```python
from build123d import *

# Parameters (mm, degrees)
SKETCH1_R           = 62.5
BOSS_EXTRUDE1_DEPTH = 25
SKETCH3_W           = 40
SKETCH3_H           = 21
SKETCH7_R           = 6.05
CUT_EXTRUDE1_DEPTH  = 205.205778567
SCALE1_SCALE        = 0.25


with BuildPart() as part:
    # Sketch1 → Boss-Extrude1 (new, symmetric)
    with BuildSketch(Plane(origin=(0, 0, 0), x_dir=(1, 0, 0), z_dir=(0, 1, 0))):
        with BuildLine():
            Line((102.443626017, 46.492510026), (95.514529523, 43.622384283))
            Line((95.514529523, 43.622384283), (98.384655266, 36.693287789))
            Line((98.384655266, 36.693287789), (105.31375176, 39.563413532))
            ThreePointArc((105.31375176, 39.563413532), (110.313875085, 22.070318614), (112.4288664, 4))
            Line((112.4288664, 4), (140, 4))
            Line((140, 4), (140, -4))
            Line((140, -4), (112.4288664, -4))
            ThreePointArc((112.4288664, -4), (110.313875085, -22.070318614), (105.31375176, -39.563413532))
            Line((105.31375176, -39.563413532), (98.384655266, -36.693287789))
            Line((98.384655266, -36.693287789), (95.514529523, -43.622384283))
            Line((95.514529523, -43.622384283), (102.443626017, -46.492510026))
            ThreePointArc((102.443626017, -46.492510026), (93.609761087, -62.397617177), (82.327640957, -76.670786708))
            Line((82.327640957, -76.670786708), (101.823376491, -96.166522241))
            Line((101.823376491, -96.166522241), (96.166522241, -101.823376491))
            Line((96.166522241, -101.823376491), (76.670786708, -82.327640957))
            ThreePointArc((76.670786708, -82.327640957), (62.397617177, -93.609761087), (46.492510026, -102.443626017))
            Line((46.492510026, -102.443626017), (43.622384283, -95.514529523))
            Line((43.622384283, -95.514529523), (36.693287789, -98.384655266))
            Line((36.693287789, -98.384655266), (39.563413532, -105.31375176))
            ThreePointArc((39.563413532, -105.31375176), (22.070318614, -110.313875085), (4, -112.4288664))
            Line((4, -112.4288664), (4, -140))
            Line((4, -140), (-4, -140))
            Line((-4, -140), (-4, -112.4288664))
            ThreePointArc((-4, -112.4288664), (-22.070318614, -110.313875085), (-39.563413532, -105.31375176))
            Line((-39.563413532, -105.31375176), (-36.693287789, -98.384655266))
            Line((-36.693287789, -98.384655266), (-43.622384283, -95.514529523))
            Line((-43.622384283, -95.514529523), (-46.492510026, -102.443626017))
            ThreePointArc((-46.492510026, -102.443626017), (-62.397617177, -93.609761087), (-76.670786708, -82.327640957))
            Line((-76.670786708, -82.327640957), (-96.166522241, -101.823376491))
            Line((-96.166522241, -101.823376491), (-101.823376491, -96.166522241))
            Line((-101.823376491, -96.166522241), (-82.327640957, -76.670786708))
            ThreePointArc((-82.327640957, -76.670786708), (-93.609761087, -62.397617177), (-102.443626017, -46.492510026))
            Line((-102.443626017, -46.492510026), (-95.514529523, -43.622384283))
            Line((-95.514529523, -43.622384283), (-98.384655266, -36.693287789))
            Line((-98.384655266, -36.693287789), (-105.31375176, -39.563413532))
            ThreePointArc((-105.31375176, -39.563413532), (-110.313875085, -22.070318614), (-112.4288664, -4))
            Line((-112.4288664, -4), (-140, -4))
            Line((-140, -4), (-140, 4))
            Line((-140, 4), (-112.4288664, 4))
            ThreePointArc((-112.4288664, 4), (-110.313875085, 22.070318614), (-105.31375176, 39.563413532))
            Line((-105.31375176, 39.563413532), (-98.384655266, 36.693287789))
            Line((-98.384655266, 36.693287789), (-95.514529523, 43.622384283))
            Line((-95.514529523, 43.622384283), (-102.443626017, 46.492510026))
            ThreePointArc((-102.443626017, 46.492510026), (-93.609761087, 62.397617177), (-82.327640957, 76.670786708))
            Line((-82.327640957, 76.670786708), (-101.823376491, 96.166522241))
            Line((-101.823376491, 96.166522241), (-96.166522241, 101.823376491))
            Line((-96.166522241, 101.823376491), (-76.670786708, 82.327640957))
            ThreePointArc((-76.670786708, 82.327640957), (-62.397617177, 93.609761087), (-46.492510026, 102.443626017))
            Line((-46.492510026, 102.443626017), (-43.622384283, 95.514529523))
            Line((-43.622384283, 95.514529523), (-36.693287789, 98.384655266))
            Line((-36.693287789, 98.384655266), (-39.563413532, 105.31375176))
            ThreePointArc((-39.563413532, 105.31375176), (-22.070318614, 110.313875085), (-4, 112.4288664))
            Line((-4, 112.4288664), (-4, 140))
            Line((-4, 140), (4, 140))
            Line((4, 140), (4, 112.4288664))
            ThreePointArc((4, 112.4288664), (22.070318614, 110.313875085), (39.563413532, 105.31375176))
            Line((39.563413532, 105.31375176), (36.693287789, 98.384655266))
            Line((36.693287789, 98.384655266), (43.622384283, 95.514529523))
            Line((43.622384283, 95.514529523), (46.492510026, 102.443626017))
            ThreePointArc((46.492510026, 102.443626017), (62.397617177, 93.609761087), (76.670786708, 82.327640957))
            Line((76.670786708, 82.327640957), (96.166522241, 101.823376491))
            Line((96.166522241, 101.823376491), (101.823376491, 96.166522241))
            Line((101.823376491, 96.166522241), (82.327640957, 76.670786708))
            ThreePointArc((82.327640957, 76.670786708), (93.609761087, 62.397617177), (102.443626017, 46.492510026))
        make_face()
        with Locations(Location((0, 0, 0), (0, 0, 270))):
            Circle(SKETCH1_R, mode=Mode.SUBTRACT)
    extrude(amount=BOSS_EXTRUDE1_DEPTH, both=True)

    # Sketch3 → Cut-Revolve1 (revolve, cut)
    with BuildSketch(Plane.XY, mode=Mode.PRIVATE) as cut_revolve1_sk:
        with Locations((-82.5, -14.5)):
            Rectangle(SKETCH3_W, SKETCH3_H)
    revolve(cut_revolve1_sk.sketch.rotate(Axis((0, 65.266274402, 0), (0, -1, 0)), 270), axis=Axis((0, 65.266274402, 0), (0, -1, 0)), mode=Mode.SUBTRACT)

    # Sketch7 → Cut-Extrude1 (cut, through all)
    with BuildSketch(Plane(origin=(0, 25, 0), x_dir=(1, 0, 0), z_dir=(0, 1, 0))):
        with Locations(Location((0, 90, 0), (0, 0, 270))):
            Circle(SKETCH7_R)
        with Locations(Location((63.639610307, 63.639610307, 0), (0, 0, 270))):
            Circle(SKETCH7_R)
        with Locations(Location((90, 0, 0), (0, 0, 270))):
            Circle(SKETCH7_R)
        with Locations(Location((63.639610307, -63.639610307, 0), (0, 0, 270))):
            Circle(SKETCH7_R)
        with Locations(Location((0, -90, 0), (0, 0, 270))):
            Circle(SKETCH7_R)
        with Locations(Location((-63.639610307, -63.639610307, 0), (0, 0, 270))):
            Circle(SKETCH7_R)
        with Locations(Location((-90, 0, 0), (0, 0, 270))):
            Circle(SKETCH7_R)
        with Locations(Location((-63.639610307, 63.639610307, 0), (0, 0, 270))):
            Circle(SKETCH7_R)
    extrude(amount=-CUT_EXTRUDE1_DEPTH, mode=Mode.SUBTRACT)


with BuildPart() as part_1:
    # Scale1: scaled about (0, 6.17055907, 0)
    add(part.part.scale(SCALE1_SCALE).moved(Location((0, 4.627919303, 0))))


solid = part_1.part
```
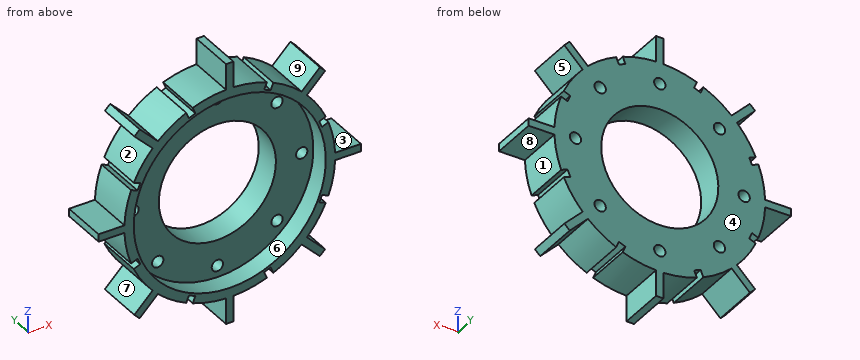
Verification items for the finished model (mm, model axes). Face numbers are marked on the shaded views. A direction names the side the tool comes from. Give positions to 0.01 mm unless a question says otherwise; leave off trailing zeros. Order: outer loops, then holes, each group sorted by start corner. A loop starts at its lowest first (then second) coordinate and runs counter-clockwise, first axis right, second up. Notation, with made-up numbers: (-36, 17.5) - (-24, 17.5) arc R34 ccw to (-24, 49.5) - close; hole circle Ø2 at (56, 73). An arc over 180 degrees is marked (long way). Answer as CSV lines item,"result". Start each with the question number.
Item 1: Access from +Z, -Z, +X, -X, +Y, -Y to the whole of each face (thin tool, end or side, straight path). Record for the marked faces 5, 6, 7, 8 and 9.
Item 2: Section check D-D, the plane y = 6. State how many separate pieces and enclosed holes the cut face has, plus the area to 3 significant figures.
Item 3: Section check A-A, the plane z = 0. Record the boundary of the cut face in (x, y) (1 decimal).
Item 4: Material ranges on L1, parallel to X at y = 6.75, z = 0 (1 decimal); L2, parallel to Z at x = -9.5, y = 7; L3, parallel to X at y = 6, z = 22.5 (1 decimal), recorded low to high.
Item 5: Section check B-B, the plane x = 0. Record the boundary of the cut face in (y, z) (1 decimal).
Item 6: Section check C-C, the plane x = -13. Record the boundary of the cut face in (y, z), plus the area to 3 significant figures.
Item 7: Mould release check, pull along Z, two halves, no side actions. Record for the marked faces 1, 2, 3 and 4: released by +Z, released by -Z, zero draft, split by the parting line, or undercut.
Item 8: Gauge pin test, flat ends, axial feed: pin 1 (7.5 mm diameter, centred on x = -32, y = 4.5, fed in from -Z); pin 2 (2 mm diameter, centred on y = 2.5, z = 30.5, fed in from +X); pin 3 (6 mm diameter, centred on y = 0.5, z = 20.5, fed in from -X). Record the tip position at first contact, or that the pin passes through.
Filled in:
1,face 5,"+X, +Y, -Y"
1,face 6,"-Y"
1,face 7,"-X, +Y, -Y"
1,face 8,"-Z, +X, +Y, -Y"
1,face 9,"+Z, +Y, -Y"
2,separate pieces,"1"
2,enclosed holes,"9"
2,area,"1,740 mm^2"
3,outline,"(-35, -1.6) - (-25.6, -1.6) - (-25.6, 3.6) - (-24, 3.6) - (-24, 10.9) - (-35, 10.9) - close; (-21, 3.6) - (-15.6, 3.6) - (-15.6, 10.9) - (-21, 10.9) - close; (15.6, 3.6) - (21, 3.6) - (21, 10.9) - (15.6, 10.9) - close; (24, 3.6) - (25.6, 3.6) - (25.6, -1.6) - (35, -1.6) - (35, 10.9) - (24, 10.9) - close"
4,L1,"-35 to -24, -21 to -15.6, 15.6 to 21, 24 to 35"
4,L2,"-26.47 to -25.38, -24.46 to -12.41, 12.41 to 24.46, 25.38 to 26.47"
4,L3,"-23.9 to -21.1, -16.9 to -1.5, 1.5 to 16.9, 21.1 to 23.9"
5,outline,"(-1.6, -35) - (10.9, -35) - (10.9, -24) - (3.6, -24) - (3.6, -25.6) - (-1.6, -25.6) - close; (-1.6, 25.6) - (3.6, 25.6) - (3.6, 24) - (10.9, 24) - (10.9, 35) - (-1.6, 35) - close; (3.6, -21) - (10.9, -21) - (10.9, -15.6) - (3.6, -15.6) - close; (3.6, 15.6) - (10.9, 15.6) - (10.9, 21) - (3.6, 21) - close"
6,outline,"(-1.62, -24.94) - (10.88, -24.94) - (10.88, -8.67) - (3.63, -8.67) - (3.63, -22.08) - (-1.62, -22.08) - close; (-1.62, 22.08) - (3.63, 22.08) - (3.63, 8.67) - (10.88, 8.67) - (10.88, 24.94) - (-1.62, 24.94) - close"
6,area,"266 mm^2"
7,face 1,"released by -Z"
7,face 2,"undercut"
7,face 3,"released by +Z"
7,face 4,"zero draft"
8,pin 1,"z = -1"
8,pin 2,"x = 1"
8,pin 3,"x = -24.91"
